from build123d import *

# Parameters (mm, degrees)
F0_W     = 26
F0_H     = 20
F1_DEPTH = 10
F2_W     = 18
F2_H     = 5
F3_DEPTH = 18
F4_W     = 26
F4_H     = 5
F5_DEPTH = 1.1
F6_R     = 0.5
F7_R     = 0.5
F8_SIZE  = 1
F10_D    = 1.75
F12_D    = 1.75
F14_D    = 2


with BuildPart() as f1:
    # F0 (on Top) → F1 (new body)
    with BuildSketch(Plane.XY):
        Rectangle(F0_W, F0_H)
    extrude(amount=F1_DEPTH)

    # F2 (on face) → F3 (cut)
    with BuildSketch(Plane(origin=(0, 10, 0), x_dir=(-1, 0, 0), z_dir=(0, 1, 0))):
        with Locations((0, 2.5)):
            Rectangle(F2_W, F2_H)
    extrude(amount=-F3_DEPTH, mode=Mode.SUBTRACT)

    # F4 (on face) → F5 (cut)
    with BuildSketch(Plane(origin=(0, 10, 0), x_dir=(-1, 0, 0), z_dir=(0, 1, 0))):
        with Locations((0, 2.5)):
            Rectangle(F4_W, F4_H)
    extrude(amount=-F5_DEPTH, mode=Mode.SUBTRACT)

    # F6
    f6_edges = [f1.edges().sort_by_distance(p)[0] for p in [
        (9, -8, 2.5),
        (-9, -8, 2.5),
        (0, -8, 5),
    ]]
    fillet(f6_edges, radius=F6_R)

    # F7
    f7_edges = [f1.edges().sort_by_distance(p)[0] for p in [
        (-11, 8.9, 5),
        (11, 8.9, 5),
    ]]
    fillet(f7_edges, radius=F7_R)

    # F8
    f8_edges = [f1.edges().sort_by_distance(p)[0] for p in [
        (13, -10, 5),
        (-13, -10, 5),
    ]]
    chamfer(f8_edges, length=F8_SIZE)

    # F10 (through all)
    with Locations(Plane(origin=(0, 8.9, 0), x_dir=(-1, 0, 0), z_dir=(0, 1, 0))):
        with Locations((-11.2, 2), (11.2, 2)):
            Hole(F10_D / 2)

    # F12 (through all)
    with Locations(Plane(origin=(-13, 0, 0), x_dir=(0, -1, 0), z_dir=(-1, 0, 0))):
        with Locations((0, 7.5)):
            Hole(F12_D / 2)

    # F14 (through all)
    with Locations(Plane.XY.offset(10)):
        with Locations((0, 0)):
            Hole(F14_D / 2)


solid = f1.part
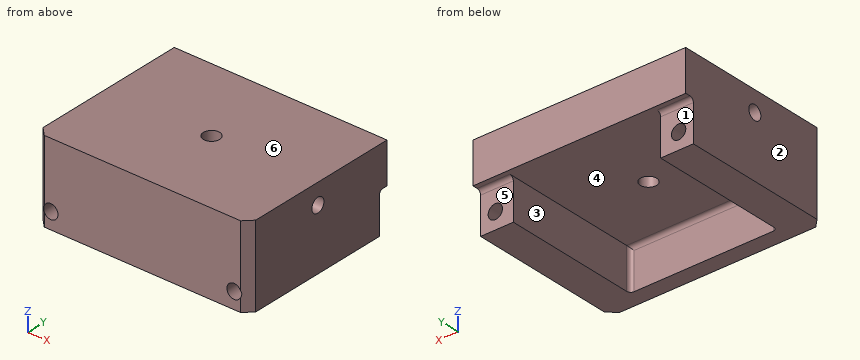
Could you check a few things on this model? Use its own coordinates, in mm. Face numbers are marked on the shaded views. A direction names the side the tool comes from. Round coordinates to 2 decimals unless told otherwise and drop trailing zeros. Loops run counter-clockwise (first coordinate to the right, second up) from the corner with the lowest first, then second, coordinate; pieces in that order, holes last. Notation, with made-up numbers: (-37, 36) -> (-26, 36) arc R23 cw to (-26, 56) -> close; hole circle Ø1 at (55.25, 20). An arc over 180 degrees is marked (long way). Use CSV: the item, a comma, the result in double quotes.
(1) If I drill on probe 1 along X at (y, z) = (-5.5, 3.25); probe 2 along X at (y, z) = (3.25, 1.25); probe 3 along Y at (x, z) = (-8.75, 7.5) (3 decimals), over which ranges is the centre line in solid material (lowest first)? Write a range as [from, to].
Return value:
probe 1,"x = [-13, -9], [9, 13]"
probe 2,"x = [-13, -11.65], [-10.75, -9], [9, 10.75], [11.65, 13]"
probe 3,"y = [-10, -0.875], [0.875, 10]"
(2) Will these pins go through, and if not, where does the flat tip stop? pin 1 Ø8 at (x, y) = (4, 4.5) entering from -Z; pin 2 Ø3 at (y, z) = (0, 7.5) entering from -X; pin 3 Ø1.8 at (x, y) = (0, 0) entering from +Z; pin 4 Ø3 at (x, z) = (10.5, 3) entering from +Y.
Return value:
pin 1,"stops at z = 5"
pin 2,"stops at x = -13"
pin 3,"passes through"
pin 4,"stops at y = 8.9"
(3) If we mould it in two halves opening along X, with no side actions, what happens to the marked faces 1, 2 and 3? For each: +X half, -X half, draft (parallel to the pull), parting line (faces both ways), or undercut.
Return value:
face 1,"draft"
face 2,"-X half"
face 3,"undercut"
(4) Suppose I cut it at C-C on z = 7.5. Write out the boundary of the cut face in (x, y) (3 decimals).
Return value:
outline,"(-13, -9) -> (-12, -10) -> (12, -10) -> (13, -9) -> (13, -0.875) -> (0.484, -0.875) arc R1 cw to (-0.484, -0.875) -> (-13, -0.875) -> close; (-13, 0.875) -> (-0.484, 0.875) arc R1 cw to (0.484, 0.875) -> (13, 0.875) -> (13, 10) -> (-13, 10) -> close"
(5) Suppose I cut it at D-D on x = 3. Write out the boundary of the cut face in (y, z) (3 decimals).
Return value:
outline,"(-10, 0) -> (-8, 0) -> (-8, 4.5) arc R0.5 cw to (-7.5, 5) -> (10, 5) -> (10, 10) -> (-10, 10) -> close; hole circle Ø1.75 at (0, 7.5)"
(6) Suppose I cut it at A-A on y = 0. Write out the boundary of the cut face in (x, z) (3 decimals), plus the area to 3 significant figures.
Return value:
outline,"(-13, 0) -> (-9, 0) -> (-9, 5) -> (-1, 5) -> (-1, 6.625) -> (-13, 6.625) -> close; (-13, 8.375) -> (-1, 8.375) -> (-1, 10) -> (-13, 10) -> close; (1, 5) -> (9, 5) -> (9, 0) -> (13, 0) -> (13, 6.625) -> (1, 6.625) -> close; (1, 8.375) -> (13, 8.375) -> (13, 10) -> (1, 10) -> close; hole circle Ø1.75 at (-11.2, 2); hole circle Ø1.75 at (11.2, 2)"
area,"113 mm²"
(7) For the marked faces 4, 5 and 6, which set-ups out of +Z, -Z, +X, -X, +Y, -Y let a thin tool reach every point of the face, with its end or its side?
Return value:
face 4,"-Z, +Y"
face 5,"-Z, +X, -X, +Y"
face 6,"+Z, +X, -X, +Y, -Y"
(8) Suppose I cut it at B-B on x = -11.2. Write out the boundary of the cut face in (y, z) (3 decimals).
Return value:
outline,"(-10, 0) -> (8.9, 0) -> (8.9, 1.125) -> (-10, 1.125) -> close; (-10, 2.875) -> (8.9, 2.875) -> (8.9, 4.5) arc R0.5 cw to (9.4, 5) -> (10, 5) -> (10, 10) -> (-10, 10) -> close; hole circle Ø1.75 at (0, 7.5)"
